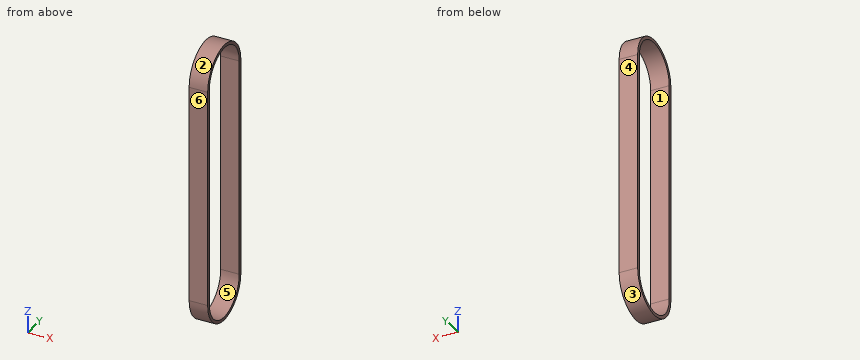
from build123d import *

# Parameters (mm, degrees)
EXTRUDE_THIN1_DEPTH = 3


with BuildPart() as part:
    # Sketch1 → Extrude-Thin1 (new, symmetric)
    with BuildSketch(Plane(origin=(0, 0, 0), x_dir=(0, 0, -1), z_dir=(1, 0, 0))):
        with BuildLine():
            Line((-71.545, 10.33), (0, 10.33))
            ThreePointArc((0, 10.33), (10.33, 0), (0, -10.33))
            Line((0, -10.33), (-71.545, -10.33))
            ThreePointArc((-71.545, -10.33), (-81.875, 0), (-71.545, 10.33))
        make_face()
        with BuildLine():
            Line((-71.545, 9.33), (0, 9.33))
            ThreePointArc((0, 9.33), (9.33, 0), (0, -9.33))
            Line((0, -9.33), (-71.545, -9.33))
            ThreePointArc((-71.545, -9.33), (-80.875, 0), (-71.545, 9.33))
        make_face(mode=Mode.SUBTRACT)
    extrude(amount=EXTRUDE_THIN1_DEPTH, both=True)


solid = part.part
Geometry: final body of the model. Coordinates: model frame, mm. Face numbers are marked on the shaded views. A direction names the side the tool comes from. Coordinates: 2 decimals unless noted, no trailing zeros. Write each loop counter-clockwise with the first axis right and the second up, starting at its lowest first coordinate (ties: lowest second). Pieces come first, ordered by that corner, then holes. Notation, with made-up numbers: (-28.5, 87.25) - (7.5, 87.25) arc R34 ccw to (7.5, 122.25) - close; hole circle Ø1 at (-13, 43.5). An arc over 180 degrees is marked (long way). Return JSON: item names as keys, results as strings.
Item 1: Pull-direction query (Y, two-part tool) for the marked faces 3, 4, 5 and 6; classes: +Y half, -Y half, draft (parallel to the pull), parting line (faces both ways), or undercut.
Completed:
{"face 3": "parting line", "face 4": "+Y half", "face 5": "undercut", "face 6": "-Y half"}
Item 2: Line query: L1, parallel to Y at x = 2.45, z = 3; L2, parallel to Z at x = 0.2, y = 0.5; L3, parallel to Z at x = 2.2, y = -1. Output: solid intervals per line, ascending.
Completed:
{"L1": "y = -10.33 to -9.33, 9.33 to 10.33", "L2": "z = -10.32 to -9.32, 80.86 to 81.86", "L3": "z = -10.28 to -9.28, 80.82 to 81.83"}
Item 3: Pin query (flat end, axial travel): pin 1 Ø1 at (x, y) = (-2, 1.5) entering from -Z. Return the tip coordinate at first contact, or that it passes through.
Completed:
{"pin 1": "stops at z = -10.28"}
Item 4: Section query B-B (x = 1.75). Output: boundary loops of the cut face in (y, z) (3 decimals), and give its area (3 significant figures).
Completed:
{"outline": "(-10.33, 0) arc R10.33 ccw to (10.33, 0) - (10.33, 71.545) arc R10.33 ccw to (-10.33, 71.545) - close; hole (-9.33, 0) arc R9.33 ccw to (9.33, 0) - (9.33, 71.545) arc R9.33 ccw to (-9.33, 71.545) - close", "area": "205 mm2"}
Item 5: Section query C-C (y = 0). Output: boundary loops of the cut face in (x, z) (3 decimals).
Completed:
{"outline": "(-3, -10.33) - (3, -10.33) - (3, -9.33) - (-3, -9.33) - close; (-3, 80.875) - (3, 80.875) - (3, 81.875) - (-3, 81.875) - close"}
Item 6: Reachability of the marked faces 1 and 2 from +Z, -Z, +X, -X, +Y, -Y: full face, straight path, thin tool, end or side. Return the list, or none.
Completed:
{"face 1": "+X, -X", "face 2": "+Z, +X, -X"}
Item 7: Section query A-A (z = 11). Output: boundary loops of the cut face in (x, y).
Completed:
{"outline": "(-3, -10.33) - (3, -10.33) - (3, -9.33) - (-3, -9.33) - close; (-3, 9.33) - (3, 9.33) - (3, 10.33) - (-3, 10.33) - close"}
